Input: dimensioned drawing with shaded views. Units: mm. Origin: part minimum x, y, z. A direction names the side the tool comes from. Give positions to 0.01 mm unless a question says otherwise; leave off trailing zeros. Loops run counter-clockwise (first coordinate to the right, second up) from the corner with the lowest first, then second, coordinate; pieces in that order, holes last.
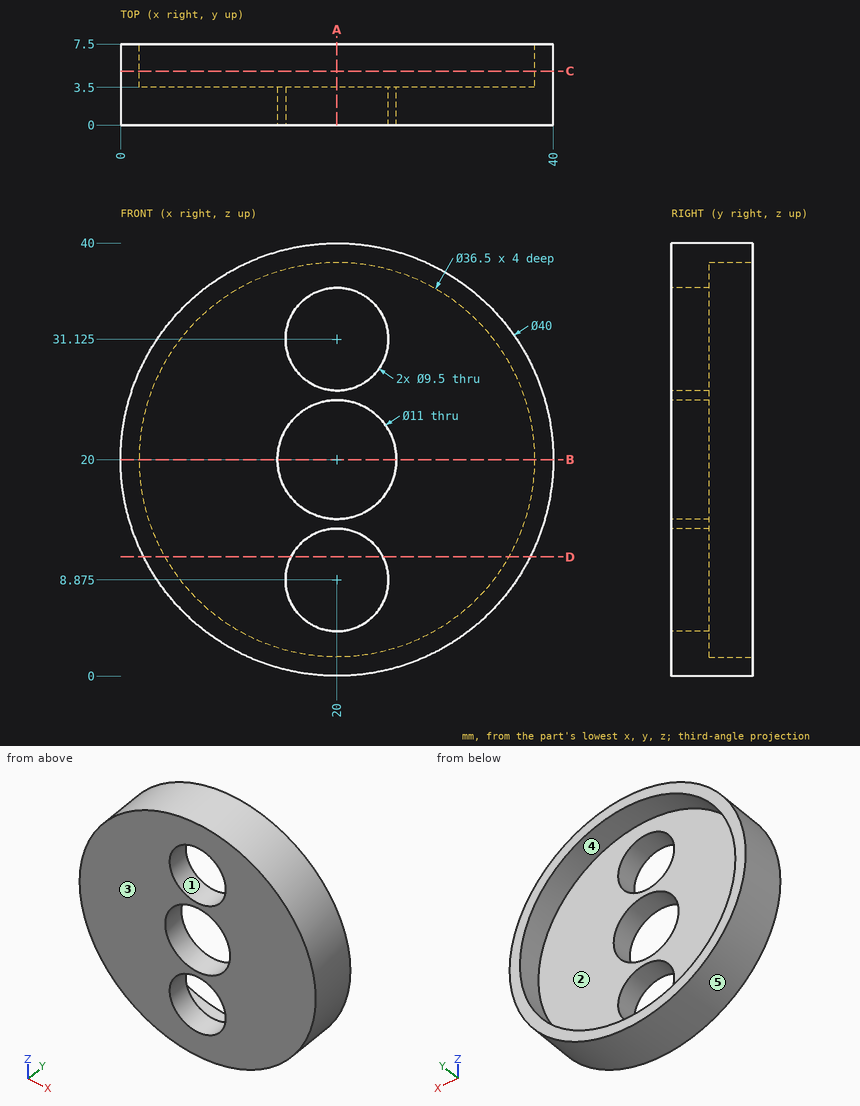
(1) Section D-D, the plane z = 11. Return the cut outline in (x, y).
A:
outline: (2.14, 0) - (15.75, 0) - (15.75, 3.5) - (4.12, 3.5) - (4.12, 7.5) - (2.14, 7.5) - close; (24.25, 0) - (37.86, 0) - (37.86, 7.5) - (35.88, 7.5) - (35.88, 3.5) - (24.25, 3.5) - close
(2) Section B-B, the plane z = 20. Return the cut outline in (x, y), then the cut area to 4 significant figures.
A:
outline: (0, 0) - (14.5, 0) - (14.5, 3.5) - (1.75, 3.5) - (1.75, 7.5) - (0, 7.5) - close; (25.5, 0) - (40, 0) - (40, 7.5) - (38.25, 7.5) - (38.25, 3.5) - (25.5, 3.5) - close
area: 115.5 mm2
(3) Section A-A, the plane x = 20. Return the cut outline in (y, z) (3 decimals).
A:
outline: (0, 0) - (7.5, 0) - (7.5, 1.75) - (3.5, 1.75) - (3.5, 4.125) - (0, 4.125) - close; (0, 13.625) - (3.5, 13.625) - (3.5, 14.5) - (0, 14.5) - close; (0, 25.5) - (3.5, 25.5) - (3.5, 26.375) - (0, 26.375) - close; (0, 35.875) - (3.5, 35.875) - (3.5, 38.25) - (7.5, 38.25) - (7.5, 40) - (0, 40) - close
(4) Ray query, line 1 along Z through (x, y) = (20, 1.4) (3 decimals); line 2 along X through (y, z) = (5.5, 20); line 3 along Z through (x, y) = (22, 3.25). Return the intervals inside material, ascending.
A:
line 1: z = 0 to 4.125, 13.625 to 14.5, 25.5 to 26.375, 35.875 to 40
line 2: x = 0 to 1.75, 38.25 to 40
line 3: z = 0.1 to 4.57, 13.18 to 14.88, 25.12 to 26.82, 35.43 to 39.9
(5) Reachability of the marked faces 1 and 2 from +Z, -Z, +X, -X, +Y, -Y: full face, straight path, thin tool, end or side. Return the list, or none.
A:
face 1: +Y, -Y
face 2: +Y
(6) Section C-C, the plane y = 5. Return the cut outline in (x, z), then the cut area to 3 significant figures.
A:
outline: circle Ø40 at (20, 20); hole circle Ø36.5 at (20, 20)
area: 210 mm2
(7) Mould query, pull axis Z, two halves, no side actions, for the marked faces 3, 4 and 5. Classes: pulls with the +Z half, pulls with the -Z half, needs draft (parallel to the pull), parting line crosses it, or undercut.
A:
face 3: needs draft
face 4: undercut
face 5: parting line crosses it
(8) First-contact query: pin 1 (8.5 mm diameter, centred on x = 20, z = 8.875, fed in from +Y); pin 2 (11 mm diameter, centred on x = 18.5, z = 24, fed in from +Y); pin 3 (1.5 mm diameter, centred on y = 1.5, z = 34, fed in from +X); pin 4 (4 mm diameter, centred on y = 3, z = 17, fed in from +X) (3 decimals). Flat tips, straight axial feed; report the tip coordinate or a pass-through.
A:
pin 1: passes through
pin 2: stops at y = 3.5
pin 3: stops at x = 34.98
pin 4: stops at x = 39.975
